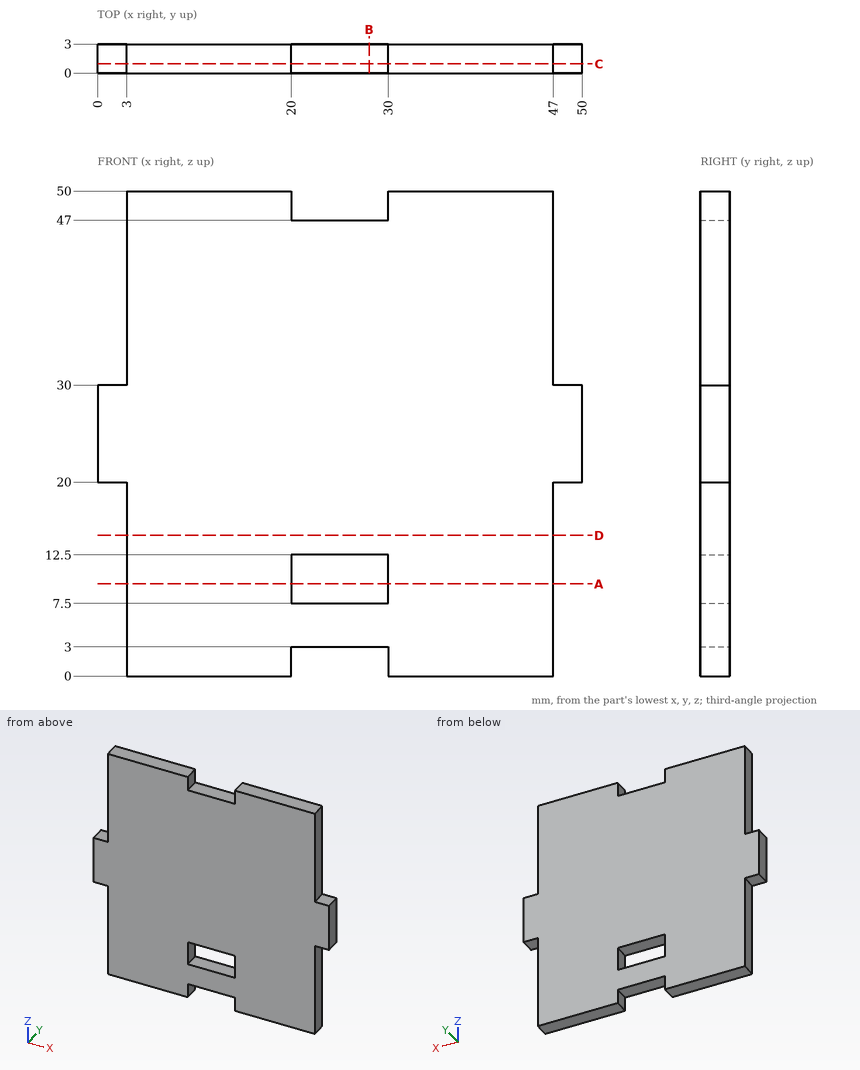
The figure shows three views and two pictorial views of one solid part (mm, origin at its lowest corner). Answer the questions. Coordinates: 2 decimals unless noted, no trailing zeros. Write each loop counter-clockwise with the first axis right and the second up, starting at its lowest first coordinate (ties: lowest second). Pieces come first, ordered by that corner, then holes.
1. The part is cut by section A-A, the plane z = 9.5. Write down the section's boundary in (x, y), and give its area (3 significant figures).
Results list:
outline: (3, 0) - (20, 0) - (20, 3) - (3, 3) - close; (30, 0) - (47, 0) - (47, 3) - (30, 3) - close
area: 102 mm2
2. Consider line 1 along Z through (x, y) = (23.5, 1.2); line 2 along X through (y, z) = (2.6, 11.5); line 3 along X through (y, z) = (1.2, 6). Determine where each line is inside the solid, lowest interval first.
Results list:
line 1: z = 3 to 7.5, 12.5 to 47
line 2: x = 3 to 20, 30 to 47
line 3: x = 3 to 47
3. Flat-ended cylindrical pins translate along their axes: pin 1 (0.9 mm diameter, centred on y = 1.5, z = 1, fed in from +X); pin 2 (1.5 mm diameter, centred on x = 27, y = 1, fed in from +Z); pin 3 (0.9 mm diameter, centred on x = 24, y = 1.5, fed in from -Z). Find the tip coordinate at first contact, or state that the pin passes through.
Results list:
pin 1: stops at x = 47
pin 2: stops at z = 47
pin 3: stops at z = 3
4. The part is cut by section C-C, the plane y = 0.95. Write down the section's boundary in (x, z).
Results list:
outline: (0, 20) - (3, 20) - (3, 0) - (20, 0) - (20, 3) - (30, 3) - (30, 0) - (47, 0) - (47, 20) - (50, 20) - (50, 30) - (47, 30) - (47, 50) - (30, 50) - (30, 47) - (20, 47) - (20, 50) - (3, 50) - (3, 30) - (0, 30) - close; hole (20, 7.5) - (30, 7.5) - (30, 12.5) - (20, 12.5) - close
5. The part is cut by section D-D, the plane z = 14.5. Write down the section's boundary in (x, y).
Results list:
outline: (3, 0) - (47, 0) - (47, 3) - (3, 3) - close
6. The part is cut by section B-B, the plane x = 28. Write down the section's boundary in (y, z).
Results list:
outline: (0, 3) - (3, 3) - (3, 7.5) - (0, 7.5) - close; (0, 12.5) - (3, 12.5) - (3, 47) - (0, 47) - close
